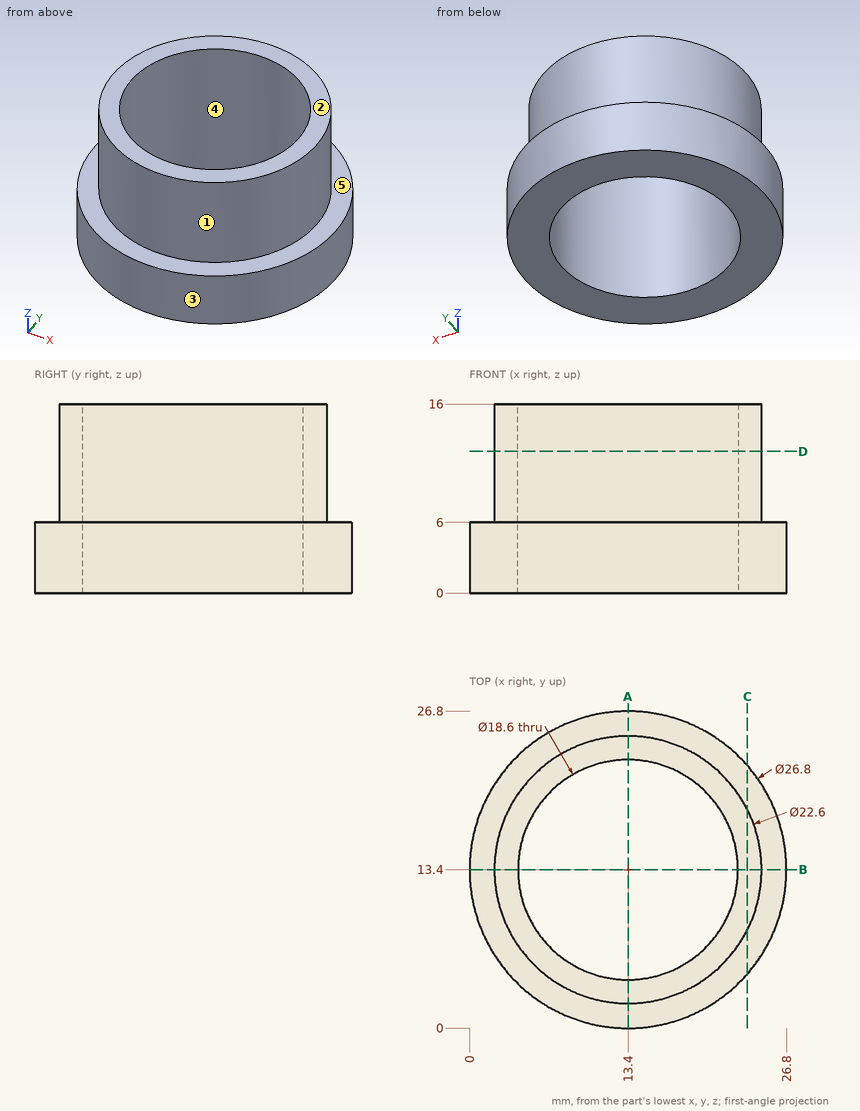
Geometry check sheet. Reference: drawing and pictorial views, mm from the part's lowest x, y, z. A direction names the side the tool comes from. Round coordinates to 2 decimals unless told otherwise and drop trailing zeros. Loops run counter-clockwise (first coordinate to the right, second up) from the corner with the lowest first, then second, coordinate; pieces in that order, holes last. Notation, with made-up numbers: (-14, 30.25) - (44, 30.25) arc R34 ccw to (44, 65.25) - close; hole circle Ø11 at (-33, 37). An arc over 180 degrees is marked (long way). Use a Markdown table: item, result. Add a question column.
1. Section check D-D, the plane z = 12. Record the boundary of the cut face in (x, y), plus the area to 3 significant figures.
2. Release check for a two-part mould opening along X. For the marked faces 3, 4 and 5 record: released by +X, released by -X, zero draft, split by the parting line, or undercut.
3. Section check C-C, the plane x = 23.5. Record the boundary of the cut face in (y, z).
4. Access from +Z, -Z, +X, -X, +Y, -Y to the whole of each face (thin tool, end or side, straight path). Record for the marked faces 1 and 2.
5. Section check A-A, the plane x = 13.4. Record the boundary of the cut face in (y, z).
6. Thickness scan on probe 1 along Y at (x, z) = (13.4, 9.5); probe 2 along Y at (x, z) = (13.4, 5); probe 3 along X at (y, z) = (11, 7.75). Record the ranges inside material, lowest first. Write a range as [from, to].
7. Gauge pin test, flat ends, axial feed: pin 1 (5 mm diameter, centred on y = 22.5, z = 1.5, fed in from -X); pin 2 (1.5 mm diameter, centred on y = 21, z = 4, fed in from -X); pin 3 (4 mm diameter, centred on y = 10, z = 7.5, fed in from -X). Record the tip position at first contact, or that the pin passes through.
Checks:
| question | item | result |
|---|---|---|
| 1 | outline | circle Ø22.6 at (13.4, 13.4); hole circle Ø18.6 at (13.4, 13.4) |
| 1 | area | 129 mm^2 |
| 2 | face 3 | split by the parting line |
| 2 | face 4 | undercut |
| 2 | face 5 | zero draft |
| 3 | outline | (4.59, 0) - (22.21, 0) - (22.21, 6) - (18.47, 6) - (18.47, 16) - (8.33, 16) - (8.33, 6) - (4.59, 6) - close |
| 4 | face 1 | +Z |
| 4 | face 2 | +Z, +X, -X, +Y, -Y |
| 5 | outline | (0, 0) - (4.1, 0) - (4.1, 16) - (2.1, 16) - (2.1, 6) - (0, 6) - close; (22.7, 0) - (26.8, 0) - (26.8, 6) - (24.7, 6) - (24.7, 16) - (22.7, 16) - close |
| 6 | probe 1 | y = [2.1, 4.1], [22.7, 24.7] |
| 6 | probe 2 | y = [0, 4.1], [22.7, 26.8] |
| 6 | probe 3 | x = [2.36, 4.42], [22.38, 24.44] |
| 7 | pin 1 | stops at x = 1.74 |
| 7 | pin 2 | stops at x = 1.88 |
| 7 | pin 3 | stops at x = 0.16 |
